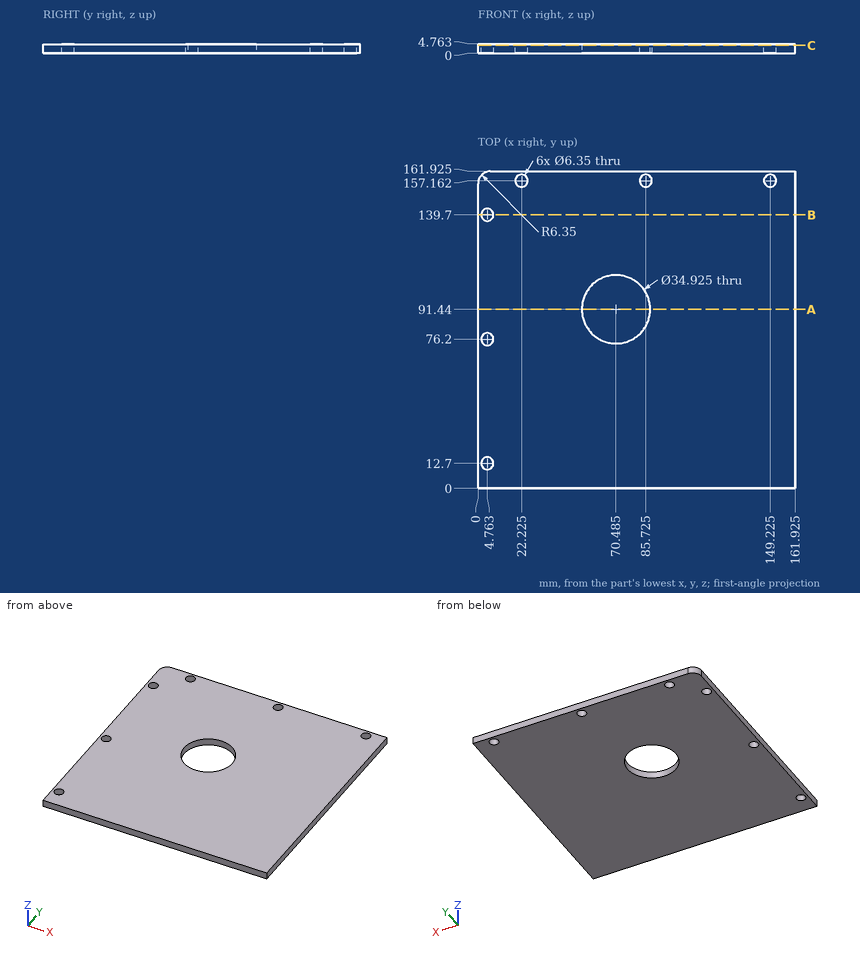
Can you work these out from the drawing? Everything is in mm from the part's minimum corner. Round coordinates to 2 decimals unless told otherwise and drop trailing zeros. Write each loop counter-clockwise with the first axis right and the second up, starting at its lowest first coordinate (ties: lowest second). Pieces come first, ordered by that corner, then holes. Notation, with made-up numbers: M -19,-34 L 31,-34 A21 cw 31,-23 Z; hole C -26,-12.75 d3. An arc over 180 degrees is marked long. Use a Markdown table: item, result.
Item 1: For pin 1 Ø21 at (x, y) = (70.485, 91.44) entering from -Z, with a flat end and sliding along its axis, tell me the tip position at first contact or that it passes through.
Found:
| item | result |
|---|---|
| pin 1 | passes through |
Item 2: I want a section at C-C (z = 4). State how many separate pieces and enclosed holes the cut face has, and give its area (3 significant figures).
Found:
| item | result |
|---|---|
| separate pieces | 1 |
| enclosed holes | 7 |
| area | 25,100 mm2 |
Item 3: I want a section at B-B (y = 139.7). List the corners of the cut face in (x, z) for me (1 decimal), and give its area (3 significant figures).
Found:
| item | result |
|---|---|
| outline | M 0,0 L 1.6,0 L 1.6,4.8 L 0,4.8 Z; M 7.9,0 L 161.9,0 L 161.9,4.8 L 7.9,4.8 Z |
| area | 741 mm2 |
Item 4: I want a section at A-A (y = 91.44). List the corners of the cut face in (x, z) for me (1 decimal).
Found:
| item | result |
|---|---|
| outline | M 0,0 L 53,0 L 53,4.8 L 0,4.8 Z; M 87.9,0 L 161.9,0 L 161.9,4.8 L 87.9,4.8 Z |
Item 5: If I drill on line 1 along X through (y, z) = (92, 3.45) (1 decimal); line 2 along X through (y, z) = (77, 0.95) (1 decimal); line 3 along Y through (x, z) = (85.5, 3.8) (1 decimal), over which ranges is the centre line in solid material (lowest first)? Write a range as [from, to].
Found:
| item | result |
|---|---|
| line 1 | x = [0, 53], [87.9, 161.9] |
| line 2 | x = [0, 1.7], [7.8, 60.7], [80.3, 161.9] |
| line 3 | y = [0, 82.5], [100.4, 154], [160.3, 161.9] |
